Work out the finished part from the listing and answer in its coordinate system (mm). A direction names the side the tool comes from. Round coordinates to 2 decimals unless told otherwise and drop trailing zeros. Write each loop counter-clockwise with the first axis right and the second up, starting at its lowest first coordinate (ties: lowest second). Pieces come first, ordered by that corner, then holes. Notation, with made-up numbers: (-2.75, -35.5) -> (5.25, -35.5) arc R26 ccw to (5.25, -17.5) -> close; hole circle Ø10 at (-36.75, -40). An arc over 180 degrees is marked (long way). One line per question, with ' | ' between items. Start each with the question number.
```python
from build123d import *

# Parameters (mm, degrees)
REVOLVE_1_ANGLE     = 180
SKETCH_2_W          = 120
SKETCH_2_H          = 124.466444362
CUT_EXTRUDE_1_DEPTH = 175.928556845
SKETCH_6_W          = 20
SKETCH_6_H          = 4.5
EXTRUDE_1_DEPTH     = 20


with BuildPart() as part:
    # Sketch 1 → Revolve 1 (revolve)
    with BuildSketch(Plane(origin=(0, 0, 0), x_dir=(0, 0, -1), z_dir=(1, 0, 0))):
        Polygon((0, 50), (0, 46), (160, 42), (160, 46), align=None)
    revolve(axis=Axis((0, 0, 0), (0, 0, -1)), revolution_arc=REVOLVE_1_ANGLE)

    # Sketch 2 → Cut-Extrude 1 (cut, through all)
    with BuildSketch(Plane(origin=(0, 0, 0), x_dir=(0, 0, -1), z_dir=(1, 0, 0))):
        with Locations((80, -2.118201403)):
            Rectangle(SKETCH_2_W, SKETCH_2_H)
    extrude(amount=CUT_EXTRUDE_1_DEPTH, mode=Mode.SUBTRACT)


with BuildPart() as cut_extrude_1_piece_1:
    # of the separate pieces the step leaves, piece 1, a body of its own (cut_extrude_1_pieces)
    add(part.part.solids().sort_by_distance((0, 50, 0))[0])



with BuildPart() as cut_extrude_1_piece_2:
    # of the separate pieces the step leaves, piece 2, a body of its own (cut_extrude_1_pieces)
    add(part.part.solids().sort_by_distance((0, 46, -160))[0])


with BuildPart() as cut_extrude_1_piece_1_1:
    add(cut_extrude_1_piece_1.part)

    add(cut_extrude_1_piece_2.part)  # Loft 1 merges Cut-Extrude 1 piece 2
    # Sketch 3 → Loft 1 section 0
    with BuildSketch(Plane.XY):
        with BuildLine():
            Line((55, 25), (45, 25))
            Line((45, 25), (45, -25))
            Line((45, -25), (55, -25))
            Line((55, -25), (55, 25))
        make_face()
    # Sketch 4 → Loft 1 section 1
    with BuildSketch(Plane(origin=(0, 0, -160), x_dir=(-1, 0, 0), z_dir=(0, 0, -1))):
        with BuildLine():
            Line((-46, 20), (-42, 20))
            Line((-42, 20), (-42, -20))
            Line((-42, -20), (-46, -20))
            Line((-46, -20), (-46, 20))
        make_face()
    loft()

    # Sketch 6 → Extrude 1 (add)
    with BuildSketch(Plane.ZY):
        with Locations((-10, 47.75)):
            Rectangle(SKETCH_6_W, SKETCH_6_H)
        with Locations((-10, -47.75)):
            Rectangle(SKETCH_6_W, SKETCH_6_H)
        with Locations((-150, -44.25)):
            Rectangle(SKETCH_6_W, SKETCH_6_H)
        with Locations((-150, 44.25)):
            Rectangle(SKETCH_6_W, SKETCH_6_H)
    extrude(amount=EXTRUDE_1_DEPTH)


solid = cut_extrude_1_piece_1_1.part
```
(1) A cutting plane is placed at A-A, the plane x = -8. Determine the outline of the cut face in (y, z).
(2) Consider L1, parallel to Y at x = -15, z = -146; L2, parallel to Z at x = 22, y = -42; L3, parallel to Y at x = 12, z = -153. Determine where each line is inside the solid, lowest interval first.
(3) Given pin 1 Ø1 at (y, z) = (-16.5, -23) entering from +X; pin 2 Ø5 at (y, z) = (-23, -64) entering from +X; pin 3 Ø0.6 at (y, z) = (42.5, -152) entering from +X, each flat-ended and moving along its own axis, determine where each tip first touches the part or whether it passes through.
(4) For faces 4 (the flat face through (-10, -50, -10)), 5 (the flat face through (-10, -42, -150)), 6 (the flat face through (-10, -46.5, -150)), determine the directions among +Z, -Z, +X, -X, +Y, -Y from which every point of the face is accessible in a straight line to the end or side of a thin tool.
(5) The mould has two halves that part along Y. Classify faces 1 (the flat face through (-10, 42, -150)), 2 (the flat face through (-10, 50, -10)), 3 (the flat face through (-20, -44, -150)): +Y half, -Y half, draft (parallel to the pull), parting line (faces both ways), or undercut.
(6) A cutting plane is placed at B-B, the plane x = 14.5. Count the separate pieces of the cut face and the enclosed holes in it, then the cut area to 3 significant figures.
Returned:
1) outline: (-50, -20) -> (-45.5, -20) -> (-45.5, 0) -> (-50, 0) -> close; (-46.5, -160) -> (-42, -160) -> (-42, -140) -> (-46.5, -140) -> close; (42, -160) -> (46.5, -160) -> (46.5, -140) -> (42, -140) -> close; (45.5, -20) -> (50, -20) -> (50, 0) -> (45.5, 0) -> close
2) L1: -46.5 to -42, 42 to 46.5 | L2: -20 to 0 | L3: -44.59 to -40.43, 40.43 to 44.59
3) pin 1: x = 53.73 | pin 2: x = 51.54 | pin 3: x = 18.8
4) face 4: +Z, -Z, +X, -X, -Y | face 5: +Z, -Z, -X | face 6: -Z, +X, -X, -Y
5) face 1: undercut | face 2: +Y half | face 3: draft
6) separate pieces: 4 | enclosed holes: 0 | area: 337 mm2
